```python
from build123d import *

# Parameters (mm, degrees)
SKETCH_1_R               = 21.6
EXTRUDE_1_DEPTH          = 4
SKETCH_6_R               = 21.45
EXTRUDE_6_DEPTH          = 21.3
SKETCH_2_R               = 2
EXTRUDE_2_DEPTH          = 15
SKETCH_3_R               = 1.25
CUT_EXTRUDE_3_DEPTH      = 3.9
PATTERN_CIRCULAR_1_COUNT = 3
SKETCH_4_R               = 6
EXTRUDE_4_DEPTH          = 3.2
EXTRUDE_START            = 7.8
SKETCH_5_R               = 2
EXTRUDE_5_DEPTH          = 7.8
SKETCH_7_R               = 21.45
SKETCH_7_R_2             = 21
CUT_EXTRUDE_7_DEPTH      = 2
EXTRUDE_9_DEPTH          = 1
CHAMFER_1_SIZE           = 0.5


with BuildPart() as part:
    # 草图1 → 拉伸1 (new body)
    with BuildSketch(Plane.XY):
        Circle(SKETCH_1_R)
    extrude(amount=EXTRUDE_1_DEPTH)

    # 草图6 → 拉伸6 (add)
    with BuildSketch(Plane(origin=(0, 0, 0), x_dir=(-1, 0, 0), z_dir=(0, 0, -1))):
        Circle(SKETCH_6_R)
    extrude(amount=-EXTRUDE_6_DEPTH)

    # 草图2 → 拉伸2 (add)
    with BuildSketch(Plane.XY.offset(21.3)):
        with Locations(Location((0, 0, 0), (0, 0, 180))):
            Circle(SKETCH_2_R)
    extrude(amount=EXTRUDE_2_DEPTH)

    # 草图3 → 拉伸3 (cut)
    with BuildSketch(Plane(origin=(0, 0, 0), x_dir=(-1, 0, 0), z_dir=(0, 0, -1))):
        with Locations((0, 11)):
            Circle(SKETCH_3_R)
    cut_extrude_3 = extrude(amount=-CUT_EXTRUDE_3_DEPTH, mode=Mode.SUBTRACT)

    # 阵列(圆周)1: 拉伸3 ×3 about axis
    pattern_circular_1_axis = Axis((0, 0, 0), (0, 0, 1))
    for i in range(1, PATTERN_CIRCULAR_1_COUNT):
        add(cut_extrude_3.rotate(pattern_circular_1_axis, i * 360 / PATTERN_CIRCULAR_1_COUNT), mode=Mode.SUBTRACT)

    # 草图4 → 拉伸4 (add)
    with BuildSketch(Plane(origin=(0, 0, 0), x_dir=(-1, 0, 0), z_dir=(0, 0, -1))):
        with Locations(Location((0, 0, 0), (0, 0, 180))):
            Circle(SKETCH_4_R)
    extrude(amount=EXTRUDE_4_DEPTH)

    # 草图5 → 拉伸5 (add)
    with BuildSketch(Plane(origin=(0, 0, -3.2), x_dir=(-1, 0, 0), z_dir=(0, 0, -1)).offset(EXTRUDE_START)):
        Circle(SKETCH_5_R)
    extrude(amount=-EXTRUDE_5_DEPTH)

    # 草图7 → 拉伸7 (cut)
    with BuildSketch(Plane.XY.offset(4)):
        with Locations(Location((0, 0, 0), (0, 0, 180))):
            Circle(SKETCH_7_R)
        Circle(SKETCH_7_R_2, mode=Mode.SUBTRACT)
    extrude(amount=CUT_EXTRUDE_7_DEPTH, mode=Mode.SUBTRACT)

    # 草图9 → 拉伸9 (add)
    with BuildSketch(Plane.XY.offset(4)):
        with BuildLine():
            Line((-10, -18.466185313), (10, -18.466185313))
            Line((10, -18.466185313), (10, -25.545340812))
            ThreePointArc((10, -25.545340812), (0, -27.432907925), (-10, -25.545340812))
            Line((-10, -25.545340812), (-10, -18.466185313))
        make_face()
    extrude(amount=EXTRUDE_9_DEPTH)

    # 倒角1
    chamfer_1_edges = [part.edges().sort_by_distance(p)[0] for p in [
        (2, 0, 36.3),
        (2, 0, -11),
    ]]
    chamfer(chamfer_1_edges, length=CHAMFER_1_SIZE)


solid = part.part
```
Source: CAD feature listing. Evaluate the final solid. Frame: model axes, mm. A direction names the side the tool comes from. Round coordinates to 2 decimals unless told otherwise and drop trailing zeros. Loops run counter-clockwise (first coordinate to the right, second up) from the corner with the lowest first, then second, coordinate; pieces in that order, holes last. Notation, with made-up numbers: M -3,22 L 45,22 A21 ccw 45,52 Z; hole C 87,61.5 d4. An arc over 180 degrees is marked long. Use a Markdown table: item, result. Add a question column.
1. Contact query for flat-ended pins moving along their axis: pin 1 (21.5 mm diameter, centred on x = -0.5, y = 6.5, fed in from -Z); pin 2 (0.8 mm diameter, centred on x = -0.5, y = 10.5, fed in from -Z); pin 3 (4 mm diameter, centred on x = -7.5, z = -6, fed in from +Y); pin 4 (3 mm diameter, centred on x = 10, z = 22, fed in from -Y). Output: stop coordinate, or through.
2. Cut plane A-A, the plane y = 0. Output: boundary loops of the cut face in (x, z), and give its area (3 significant figures).
3. Cut plane D-D, the plane z = 2.5. Output: boundary loops of the cut face in (x, y), and give its area (3 significant figures).
4. Set-up query: faces 4 (the cylindrical face through (-2.73, 20.82, 4.99)), 5 (the cylindrical face through (15.81, 14.497, 13.543)), 6 (the flat face through (0, 0, -11)), 7 (the flat face through (0, 11, 3.9)). Return all of +Z, -Z, +X, -X, +Y, -Y with unobstructed straight access to the full face (end or side cutting, diameter ignored); none if empty.
5. Ray query, line 1 along Y through (x, z) = (0, 1.35); line 2 along X through (y, z) = (-5, 2); line 3 along Z through (x, y) = (6, -17.5). Return the intervals inside material, ascending. Write a range as [from, to].
6. Pull-direction query (Y, two-part tool) for faces 1 (the flat face through (-11.3, 17.9, 4)), 2 (the flat face through (10, -6, 3.9)), 3 (the cylindrical face through (5.723, -1.802, -1.578)); classes: +Y half, -Y half, draft (parallel to the pull), parting line (faces both ways), or undercut.
7. Cut plane C-C, the plane z = 27.5. Output: boundary loops of the cut face in (x, y), and give its area (3 significant figures).
Solution:
| question | item | result |
|---|---|---|
| 1 | pin 1 | stops at z = -11 |
| 1 | pin 2 | stops at z = 3.9 |
| 1 | pin 3 | passes through |
| 1 | pin 4 | stops at y = -19.62 |
| 2 | outline | M -21.6,0 L -6,0 L -6,-3.2 L -2,-3.2 L -2,-10.5 L -1.5,-11 L 1.5,-11 L 2,-10.5 L 2,-3.2 L 6,-3.2 L 6,0 L 21.6,0 L 21.6,4 L 21,4 L 21,6 L 21.45,6 L 21.45,21.3 L 2,21.3 L 2,35.8 L 1.5,36.3 L -1.5,36.3 L -2,35.8 L -2,21.3 L -21.45,21.3 L -21.45,6 L -21,6 L -21,4 L -21.6,4 Z |
| 2 | area | 1,040 mm2 |
| 3 | outline | C 0,0 d43.2; hole C -9.53,-5.5 d2.5; hole C 0,11 d2.5; hole C 9.53,-5.5 d2.5 |
| 3 | area | 1,450 mm2 |
| 4 | face 4 | none |
| 4 | face 5 | +Z |
| 4 | face 6 | -Z, +X, -X, +Y, -Y |
| 4 | face 7 | -Z |
| 5 | line 1 | y = [-21.6, 9.75], [12.25, 21.6] |
| 5 | line 2 | x = [-21.01, -10.67], [-8.38, 8.38], [10.67, 21.01] |
| 5 | line 3 | z = [0, 21.3] |
| 6 | face 1 | draft |
| 6 | face 2 | undercut |
| 6 | face 3 | parting line |
| 7 | outline | C 0,0 d4 |
| 7 | area | 12.6 mm2 |
